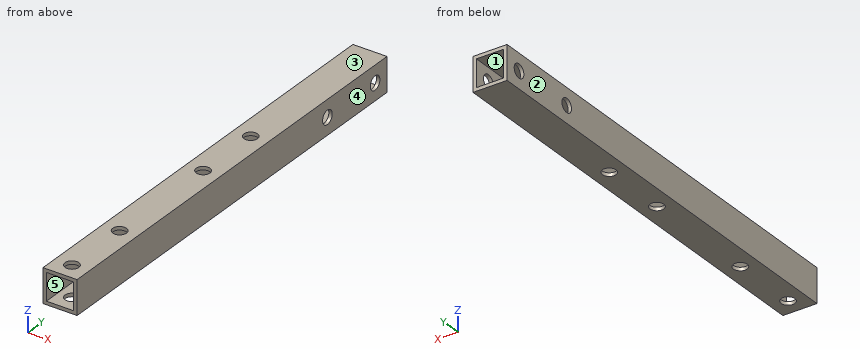
from build123d import *

# Parameters (mm, degrees)
SKETCH1_W           = 10
SKETCH1_H           = 10
SKETCH1_W_2         = 8
SKETCH1_H_2         = 8
BOSS_EXTRUDE1_DEPTH = 130
SKETCH2_R           = 2.025
CUT_EXTRUDE1_DEPTH  = 131.479883507
SKETCH3_R           = 2.025
CUT_EXTRUDE2_DEPTH  = 131.479883507
SKETCH4_R           = 2.025
CUT_EXTRUDE3_DEPTH  = 131.479883507


with BuildPart() as part:
    # Sketch1 → Boss-Extrude1 (new body)
    with BuildSketch(Plane(origin=(0, 0, 0), x_dir=(1, 0, 0), z_dir=(0, 1, 0))):
        Rectangle(SKETCH1_W, SKETCH1_H)
        Rectangle(SKETCH1_W_2, SKETCH1_H_2, mode=Mode.SUBTRACT)
    extrude(amount=BOSS_EXTRUDE1_DEPTH)

    # Sketch2 → Cut-Extrude1 (cut, through all)
    with BuildSketch(Plane.XY.offset(5)):
        with Locations((0, 5)):
            Circle(SKETCH2_R)
        with Locations((0, 25)):
            Circle(SKETCH2_R)
    extrude(amount=-CUT_EXTRUDE1_DEPTH, mode=Mode.SUBTRACT)

    # Sketch3 → Cut-Extrude2 (cut, through all)
    with BuildSketch(Plane(origin=(5, 0, 0), x_dir=(0, 0, -1), z_dir=(1, 0, 0))):
        with Locations((0, 125)):
            Circle(SKETCH3_R)
        with Locations((0, 105)):
            Circle(SKETCH3_R)
    extrude(amount=-CUT_EXTRUDE2_DEPTH, mode=Mode.SUBTRACT)

    # Sketch4 → Cut-Extrude3 (cut, through all)
    with BuildSketch(Plane.XY.offset(5)):
        with Locations((0, 60)):
            Circle(SKETCH4_R)
        with Locations((0, 80)):
            Circle(SKETCH4_R)
    extrude(amount=-CUT_EXTRUDE3_DEPTH, mode=Mode.SUBTRACT)


solid = part.part
Geometry check sheet. Reference: the model listing, model coordinates, mm. Face numbers are marked on the shaded views. A direction names the side the tool comes from. Give positions to 0.01 mm unless a question says otherwise; leave off trailing zeros. Order: outer loops, then holes, each group sorted by start corner. A loop starts at its lowest first (then second) coordinate and runs counter-clockwise, first axis right, second up.
1. Scan lines: line 1 (Y direction, x = 0, z = 4.45) (3 decimals); line 2 (Z direction, x = 1.5, y = 72). Record each from-to range of solid material in increasing order.
Completed:
line 1: y = 0 to 2.975, 7.025 to 22.975, 27.025 to 57.975, 62.025 to 77.975, 82.025 to 130
line 2: z = -5 to -4, 4 to 5
2. Sectioned sample at B-B (y = 100.5). Record the boundary of the cut face in (x, z).
Completed:
outline: (-5, -5) - (5, -5) - (5, 5) - (-5, 5) - close; hole (-4, -4) - (4, -4) - (4, 4) - (-4, 4) - close
3. Draft check along X on the marked faces 3, 4 and 5. Enter one of: pulls with the +X half, pulls with the -X half, needs draft (parallel to the pull), parting line crosses it, or undercut.
Completed:
face 3: needs draft
face 4: pulls with the +X half
face 5: undercut
4. Sectioned sample at C-C (y = 25). Record the boundary of the cut face in (x, z) (3 decimals), then the cut area to 3 significant figures.
Completed:
outline: (-5, -5) - (-2.025, -5) - (-2.025, -4) - (-4, -4) - (-4, 4) - (-2.025, 4) - (-2.025, 5) - (-5, 5) - close; (2.025, -5) - (5, -5) - (5, 5) - (2.025, 5) - (2.025, 4) - (4, 4) - (4, -4) - (2.025, -4) - close
area: 27.9 mm2
5. Access from +Z, -Z, +X, -X, +Y, -Y to the whole of each face (thin tool, end or side, straight path). Record for the marked faces 1 and 2.
Completed:
face 1: +Y, -Y
face 2: +Z, -Z, -X, +Y, -Y
6. Sectioned sample at A-A (z = 0). Record the boundary of the cut face in (x, y) (3 decimals), then the cut area to 3 significant figures.
Completed:
outline: (-5, 0) - (-4, 0) - (-4, 102.975) - (-5, 102.975) - close; (-5, 107.025) - (-4, 107.025) - (-4, 122.975) - (-5, 122.975) - close; (-5, 127.025) - (-4, 127.025) - (-4, 130) - (-5, 130) - close; (4, 0) - (5, 0) - (5, 102.975) - (4, 102.975) - close; (4, 107.025) - (5, 107.025) - (5, 122.975) - (4, 122.975) - close; (4, 127.025) - (5, 127.025) - (5, 130) - (4, 130) - close
area: 244 mm2
